from build123d import *

# Parameters (mm, degrees)
BOSS_EXTRUDE1_DEPTH     = 40
CUT_EXTRUDE1_DEPTH      = 155.819249449
CUT_EXTRUDE1_DEPTH_BACK = 155.819249449
CUT_EXTRUDE2_DEPTH      = 25
CUT_EXTRUDE3_DEPTH      = 155.819249449


with BuildPart() as part:
    # Sketch1 → Boss-Extrude1 (new body)
    with BuildSketch(Plane.XY):
        Polygon((0, 0), (60, 0), (60, 12), (50, 12), (50, 17), (60, 17), (60, 137), (0, 137), (0, 17), (10, 17), (10, 12), (0, 12), align=None)
    extrude(amount=BOSS_EXTRUDE1_DEPTH)

    # Sketch2 → Cut-Extrude1 (cut, two sides: drawn at the far end of the back side and taken through both)
    with BuildSketch(Plane(origin=(0, 0, 0), x_dir=(0, 0, -1), z_dir=(1, 0, 0)).offset(-CUT_EXTRUDE1_DEPTH_BACK)):
        Polygon((-40, 137), (-37, 137), (-40, 127.460607986), (-37, 127.460607986), (-40, 117.921215972), (-37, 117.921215972), (-40, 108.381823957), (-37, 108.381823957), (-40, 98.842431943), (-37, 98.842431943), (-40, 89.303039929), (-37, 89.303039929), (-40, 79.763647915), (-37, 79.763647915), (-40, 70.224255901), (-37, 70.224255901), (-40, 60.684863887), (-47.730210084, 60.684863887), (-47.730210084, 137), align=None)
    extrude(amount=CUT_EXTRUDE1_DEPTH + CUT_EXTRUDE1_DEPTH_BACK, mode=Mode.SUBTRACT)

    # Sketch3 → Cut-Extrude2 (cut)
    with BuildSketch(Plane(origin=(0, 0, 0), x_dir=(-1, 0, 0), z_dir=(0, 0, -1))):
        Polygon((-60, 0), (0, 0), (0, 12), (-10, 12), (-10, 17), (-50, 17), (-50, 12), (-60, 12), align=None)
    extrude(amount=-CUT_EXTRUDE2_DEPTH, mode=Mode.SUBTRACT)

    # Sketch4 → Cut-Extrude3 (cut, through all)
    with BuildSketch(Plane(origin=(0, 137, 0), x_dir=(1, 0, 0), z_dir=(0, 1, 0))):
        with BuildLine():
            Line((0, -6.193777394), (0, 6.02263776))
            Line((0, 6.02263776), (60, 6.02263776))
            Line((60, 6.02263776), (60, -6.193777394))
            ThreePointArc((60, -6.193777394), (30, 0), (0, -6.193777394))
        make_face()
    extrude(amount=-CUT_EXTRUDE3_DEPTH, mode=Mode.SUBTRACT)


solid = part.part
The listing builds one solid part. Answer for the finished solid, in the listing's coordinates (mm). A direction names the side the tool comes from. Round coordinates to 2 decimals unless told otherwise and drop trailing zeros. Order: outer loops, then holes, each group sorted by start corner. A loop starts at its lowest first (then second) coordinate and runs counter-clockwise, first axis right, second up. Notation, with made-up numbers: M 52.5,65 L 92.5,65 A24 cw 92.5,89 Z; hole C -1.5,33.5 d11. An arc over 180 degrees is marked long. Answer in a Markdown table with one row per item. Add a question column.
1) The part is cut by section B-B on z = 4. Determine the outline of the cut face in (x, y).
2) The part is cut by section A-A on x = 55.5. Determine the outline of the cut face in (y, z), plus the area to 4 significant figures.
3) The part is cut by section D-D on y = 40. Determine the outline of the cut face in (x, z), plus the area to 3 significant figures.
4) Consider line 1 along Y through (x, z) = (49, 15.5); line 2 along Z through (x, y) = (17.5, 103.5); line 3 along Z through (x, y) = (56, 51). Determine where each line is inside the solid, lowest interval first. Write a range as from..to.
5) Determine the mould class of faces 4 (the face through (0, 6, 32)), 5 (the face through (30, 137, 18)), 6 (the face through (30, 108.382, 39)) for opening direction Y: pulls with the +Y half, pulls with the -Y half, needs draft (parallel to the pull), parting line crosses it, or undercut.
6) Flat-ended cylindrical pins translate along their axes: pin 1 Ø1.5 at (y, z) = (14, 30) entering from +X; pin 2 Ø5 at (x, y) = (40, 12) entering from -Z; pin 3 Ø8 at (x, y) = (43, 30.5) entering from -Z. Find the tip coordinate at first contact, or state that the pin passes through.
7) Which of the six approach directions +Z, -Z, +X, -X, +Y, -Y give full straight-line access (tool end or side, diameter ignored) to faces 1 (the face through (30, 9, 25)), 2 (the face through (29.58, 103.68, 38.48)), 3 (the face through (5, 12, 32))?
8) The part is cut by section C-C on x = 23. Determine the outline of the cut face in (y, z), plus the area to 3 significant figures.
Findings below:
| question | item | result |
|---|---|---|
| 1 | outline | M 5.71,17 L 54.29,17 L 54.29,137 L 5.71,137 Z |
| 2 | outline | M 0,25 L 12,25 L 12,40 L 0,40 Z; M 17,4.42 L 137,4.42 L 137,37 L 127.46,40 L 127.46,37 L 117.92,40 L 117.92,37 L 108.38,40 L 108.38,37 L 98.84,40 L 98.84,37 L 89.3,40 L 89.3,37 L 79.76,40 L 79.76,37 L 70.22,40 L 70.22,37 L 60.68,40 L 17,40 Z |
| 2 | area | 4,335 mm² |
| 3 | outline | M 0,6.19 A75.75 ccw 60,6.19 L 60,40 L 0,40 Z |
| 3 | area | 2,280 mm² |
| 4 | line 1 | y = 17..137 |
| 4 | line 2 | z = 1.04..38.54 |
| 4 | line 3 | z = 4.6..40 |
| 5 | face 4 | needs draft |
| 5 | face 5 | pulls with the +Y half |
| 5 | face 6 | undercut |
| 6 | pin 1 | stops at x = 50 |
| 6 | pin 2 | stops at z = 25 |
| 6 | pin 3 | stops at z = 0.54 |
| 7 | face 1 | -Z, +X, -X, -Y |
| 7 | face 2 | +Z, +X, -X |
| 7 | face 3 | +Z, -Z, -X |
| 8 | outline | M 0,25 L 17,25 L 17,0.32 L 137,0.32 L 137,37 L 127.46,40 L 127.46,37 L 117.92,40 L 117.92,37 L 108.38,40 L 108.38,37 L 98.84,40 L 98.84,37 L 89.3,40 L 89.3,37 L 79.76,40 L 79.76,37 L 70.22,40 L 70.22,37 L 60.68,40 L 0,40 Z |
| 8 | area | 4,900 mm² |
